from build123d import *

# Parameters (mm, degrees)
F0_R      = 7.75
F0_R_2    = 7.25
F0_R_3    = 15
F0_W      = 60
F0_H      = 86.4
F1_DEPTH  = 225
F2_DEPTH  = 50
F2_TAPER  = 3
F3_DEPTH  = 50
F3_TAPER  = 3
F4_DEPTH  = 10
F5_DEPTH  = 10
F6_R      = 2.5
F7_DEPTH  = 40
F8_R      = 53
F9_DEPTH  = 97
F10_R     = 16.9998611114
F11_DEPTH = 100


with BuildPart() as f1:
    # F0 (on Front) → F1 (new body)
    with BuildSketch(Plane.XZ):
        Polygon((-72.7, -34.5117315553), (-72.7, -49.5117315553), (127.6, -49.5117315553), (127.6, -34.5117315553), (107.6, -34.5117315553), (107.6, 231.6882684447), (-52.7, 231.6882684447), (-52.7, -34.5117315553), align=None)
        with Locations((0, 97.4882684447)):
            Circle(F0_R, mode=Mode.SUBTRACT)
        with Locations((27.5, 56.4882684447)):
            Circle(F0_R_2, mode=Mode.SUBTRACT)
        with Locations((55, 56.4882684447)):
            Circle(F0_R_3, mode=Mode.SUBTRACT)
        with Locations((27.5, 97.4882684447)):
            Circle(F0_R, mode=Mode.SUBTRACT)
        with Locations((27.5, 162.2882684447)):
            Rectangle(F0_W, F0_H, mode=Mode.SUBTRACT)
        with BuildLine():
            ThreePointArc((107.6, 231.6882684447), (27.45, 248.6882684447), (-52.7, 231.6882684447))
            Line((-52.7, 231.6882684447), (107.6, 231.6882684447))
        make_face()
        with Locations((27.5, 162.2882684447)):
            Rectangle(F0_W, F0_H)
        with Locations((0, 97.4882684447)):
            Circle(F0_R)
        with Locations((27.5, 97.4882684447)):
            Circle(F0_R)
        with Locations((55, 56.4882684447)):
            Circle(F0_R_3)
        with Locations((27.5, 56.4882684447)):
            Circle(F0_R_2)
    extrude(amount=-F1_DEPTH)

    # F0 (on Front) → F2 (join)
    with BuildSketch(Plane.XZ):
        with Locations((0, 97.4882684447)):
            Circle(F0_R)
        with Locations((27.5, 97.4882684447)):
            Circle(F0_R)
    extrude(amount=F2_DEPTH, taper=F2_TAPER)

    # F0 (on Front) → F3 (join)
    with BuildSketch(Plane.XZ):
        with Locations((27.5, 56.4882684447)):
            Circle(F0_R_2)
    extrude(amount=F3_DEPTH, taper=F3_TAPER)

    # F0 (on Front) → F4 (cut)
    with BuildSketch(Plane.XZ):
        with Locations((27.5, 162.2882684447)):
            Rectangle(F0_W, F0_H)
    extrude(amount=-F4_DEPTH, mode=Mode.SUBTRACT)

    # F0 (on Front) → F5 (join)
    with BuildSketch(Plane.XZ):
        with Locations((55, 56.4882684447)):
            Circle(F0_R_3)
    extrude(amount=F5_DEPTH)

    # F6 (on face) → F7 (join)
    with BuildSketch(Plane.XZ.offset(10)):
        with Locations((55, 56.4882684447)):
            Circle(F6_R)
    extrude(amount=F7_DEPTH)

    # F8 (on face) → F9 (join)
    with BuildSketch(Plane(origin=(0, 225, 0), x_dir=(-1, 0, 0), z_dir=(0, 1, 0))):
        with Locations((-27.4, 135.6882684447)):
            Circle(F8_R)
    extrude(amount=F9_DEPTH)

    # F10 (on face) → F11 (join)
    with BuildSketch(Plane(origin=(0, 322, 0), x_dir=(-1, 0, 0), z_dir=(0, 1, 0))):
        with Locations((-27.5, 171.6882684447)):
            Circle(F10_R)
    extrude(amount=F11_DEPTH)


solid = f1.part
Part model, mm, in its own coordinate system. A direction names the side the tool comes from. Round coordinates to 2 decimals unless told otherwise and drop trailing zeros. Write each loop counter-clockwise with the first axis right and the second up, starting at its lowest first coordinate (ties: lowest second). Pieces come first, ordered by that corner, then holes. Notation, with made-up numbers: M -7,87.5 L -3,87.5 A30 cw -3,109.5 Z; hole C 79.25,38 d5. An arc over 180 degrees is marked long. Return JSON: item names as keys, results as strings. Group by question number.
(1) Which spindle directions (+Z, -Z, +X, -X, +Y, -Y) get a long thin tool onto all of the face, cutting with end or side? Do faces 4 (the face through (57.5, 5, 162)), 5 (the face through (127.6, 111, -42)), 6 (the face through (-63, 111, -34.512)), 7 (the face through (2.94, 272.82, 88.67)), 8 (the face through (118, 111, -34.512)). Say none if no direction does.
(2) Two-plate mould, pull along Z, no slides. Class faces 1 (the face through (27, 5, 205.488)), 2 (the face through (28, 322, 136)), 3 (the face through (26, 111, -49.512)): +Z half, -Z half, draft (parallel to the pull), parting line (faces both ways), or undercut.
(3) Pin check, flat tips, straight feed: pin 1 Ø8 at (y, z) = (7, 150.5) entering from +X; pin 2 Ø12 at (x, z) = (78, 79) entering from -Y; pin 3 Ø3 at (x, z) = (7.5, 186.5) entering from -Y. Stop position of each tip, or through.
(4) Saw through at C-C on y = 243. Write the cut outline in (x, z), then the cut area to 3 significant figures.
(5) Drill centre lines: probe 1 along X at (y, z) = (41.5, -21.5); probe 2 along Y at (x, z) = (89.5, 74.5); probe 3 along Y at (x, z) = (-21.5, 144.5). Where is each one in solid material? Low to high.
(6) Saw through at A-A on z = 33.5. Write the cut outline in (x, y).
(7) Saw through at B-B on x = -38.5. Write the cut outline in (y, z), then the cut area to 3 significant figures.
Returned:
{
 "1": {"face 4": "-Y", "face 5": "+Z, -Z, +X, +Y, -Y", "face 6": "+Z, -X, +Y, -Y", "face 7": "+Y", "face 8": "+Z, +X, +Y, -Y"},
 "2": {"face 1": "undercut", "face 2": "draft", "face 3": "-Z half"},
 "3": {"pin 1": "x = 107.6", "pin 2": "y = 0", "pin 3": "y = 10"},
 "4": {"outline": "C 27.4,135.69 d106", "area": "8,820 mm²"},
 "5": {"probe 1": "-52.7 to 107.6", "probe 2": "0 to 225", "probe 3": "0 to 322"},
 "6": {"outline": "M -52.7,0 L 107.6,0 L 107.6,225 L -52.7,225 Z"},
 "7": {"outline": "M 0,-49.51 L 225,-49.51 L 225,237.35 L 0,237.35 Z", "area": "64,500 mm²"}
}
